```python
from build123d import *

# Parameters (mm, degrees)
SKETCH1_W                 = 25.4
SKETCH1_H                 = 15.24
BOSS_EXTRUDE1_DEPTH       = 0.79375
EDGE_FLANGE1_DEPTH        = 25.4
F_6_START                 = -0.79375
F_6_CLEARANCE_SLOT1_DEPTH = 1.5875
M18_CLEARANCE_HOLE1_D     = 20
M18_CLEARANCE_HOLE1_DEPTH = 9.652
M18_CLEARANCE_HOLE1_TIP   = 6.00860619


# Read off the part's stored shape, not the designer's step: #6 Clearance Slot1
# Sheet-metal steps are written as plain solids
with BuildPart() as part:
    # Sketch1 → Boss-Extrude1 (new, symmetric)
    with BuildSketch(Plane.XY):
        Rectangle(SKETCH1_W, SKETCH1_H)
    extrude(amount=BOSS_EXTRUDE1_DEPTH, both=True)

    # Edge-Flange1 section (across the edge) → Edge-Flange1 (add)
    with BuildSketch(Plane(origin=(-12.7, 7.988235857, -0.79375), x_dir=(0, -0.7071067811865438, -0.7071067811865512), z_dir=(1, 0, 0))):
        with BuildLine():
            Line((-1.5875, 0.368235857), (-1.5875, 30.48))
            Line((-1.5875, 30.48), (0, 30.48))
            Line((0, 30.48), (0, 0.368235857))
            ThreePointArc((0, 0.368235857), (0.067671096, 0.028030286), (0.260382072, -0.260382072))
            Line((0.260382072, -0.260382072), (-0.862149944, -1.382914087))
            ThreePointArc((-0.862149944, -1.382914087), (-1.398987662, -0.579479663), (-1.5875, 0.368235857))
        make_face()
    extrude(amount=EDGE_FLANGE1_DEPTH)

    # #6 Clearance Slot1 outline → #6 Clearance Slot1 (cut)
    with BuildSketch(Plane.XY.offset(F_6_START)):
        with BuildLine():
            ThreePointArc((-3.24485, 3.4925), (-5.3975, 5.64515), (-7.55015, 3.4925))
            Line((-7.55015, 3.4925), (-7.55015, -3.4925))
            ThreePointArc((-7.55015, -3.4925), (-5.3975, -5.64515), (-3.24485, -3.4925))
            Line((-3.24485, -3.4925), (-3.24485, 3.4925))
        make_face()
        with BuildLine():
            ThreePointArc((3.24485, -3.4925), (5.3975, -5.64515), (7.55015, -3.4925))
            Line((7.55015, -3.4925), (7.55015, 3.4925))
            ThreePointArc((7.55015, 3.4925), (5.3975, 5.64515), (3.24485, 3.4925))
            Line((3.24485, 3.4925), (3.24485, -3.4925))
        make_face()
    extrude(amount=F_6_CLEARANCE_SLOT1_DEPTH, mode=Mode.SUBTRACT)

    # M18 Clearance Hole1
    with Locations(Plane(origin=(0, 3.597242928, 3.597242928), x_dir=(-1, 0, 0), z_dir=(0, -0.7071067811865438, -0.7071067811865512))):
        with Locations((0, 21.818037609)):
            Hole(M18_CLEARANCE_HOLE1_D / 2, depth=M18_CLEARANCE_HOLE1_DEPTH)
            with Locations((0, 0, -(M18_CLEARANCE_HOLE1_DEPTH + M18_CLEARANCE_HOLE1_TIP / 2))):  # 118° drill point
                Cone(0, M18_CLEARANCE_HOLE1_D / 2, M18_CLEARANCE_HOLE1_TIP, mode=Mode.SUBTRACT)


solid = part.part
```
Geometry: final body of the model. Coordinates: model frame, mm. A direction names the side the tool comes from. Coordinates: 2 decimals unless noted, no trailing zeros. Write each loop counter-clockwise with the first axis right and the second up, starting at its lowest first coordinate (ties: lowest second). Pieces come first, ordered by that corner, then holes. Notation, with made-up numbers: M 52,-38 L 79,-38 A21 ccw 79,1 Z; hole C -2.5,39 d6. An arc over 180 degrees is marked long. Answer as CSV lines item,"result". Start each with the question number.
Q1. Pin query (flat end, axial travel): P1, Ø4, axis at x = 1, y = 14, coming from the -Z side; P2, Ø12, axis at y = 4.5, z = -1.5, coming from the -X side; P3, Ø6, axis at x = 8.5, y = 17.5, coming from the -Z side; P4, Ø4, axis at x = 6.5, y = -2, coming from the -Z side. Return the tip coordinate at first contact, or that it passes through.
Q2. Cut plane A-A on y = 3. Return the cut outline in (x, z).
Q3. Mould query, pull axis X, two halves, no side actions, for faces 1 (the flat face through (-3, 26.141, -18.947)), 2 (the flat face through (3.245, 0, 0)), 3 (the flat face through (-12.7, 14, -6)). Classes: released by +X, released by -X, zero draft, split by the parting line, or undercut.
Q4. Cut plane C-C on x = -9. Return the cut outline in (y, z), then the cut area to 3 significant figures.
Q5. Line query: line 1 (Z direction, x = -8.5, y = 0); line 2 (Z direction, x = 4.75, y = 9.5); line 3 (Y direction, x = 4.5, z = -18.75). Output: solid intervals per line, ascending. Write a range as from..to.
Q6. Reachability of faces 4 (the flat face through (0, 0, 0.794)), 5 (the flat face through (-3.245, 0, 0)), 6 (the flat face through (0, 0, -0.794)) from +Z, -Z, +X, -X, +Y, -Y: full face, straight path, thin tool, end or side. Return the list, or none.
Q7. Cut plane B-B on x = 11.25. Return the cut outline in (y, z), then the cut area to 3 significant figures.
Q8. Cut plane D-D on x = -5.25. Return the cut outline in (y, z), then the cut area to 3 significant figures.
Findings below:
1,P1,"stops at z = -4.81"
1,P2,"stops at x = -12.7"
1,P3,"stops at z = -12.98"
1,P4,"stops at z = -0.79"
2,outline,"M -12.7,-0.79 L -7.55,-0.79 L -7.55,0.79 L -12.7,0.79 Z; M -3.24,-0.79 L 3.24,-0.79 L 3.24,0.79 L -3.24,0.79 Z; M 7.55,-0.79 L 12.7,-0.79 L 12.7,0.79 L 7.55,0.79 Z"
3,face 1,"zero draft"
3,face 2,"undercut"
3,face 3,"released by -X"
4,outline,"M -7.62,-0.79 L 7.62,-0.79 A0.89 cw 8.25,-1.05 L 15.94,-8.75 L 17.07,-7.63 L 9.37,0.07 A2.48 ccw 7.62,0.79 L -7.62,0.79 Z; M 22.11,-14.91 L 29.54,-22.35 L 30.66,-21.22 L 23.23,-13.79 Z"
4,area,"60.3 mm2"
5,line 1,"z = -0.79..0.79"
5,line 2,"z = -2.31..-0.06"
5,line 3,"y = 25.94..28.19"
6,face 4,"+Z, +X, -X, +Y, -Y"
6,face 5,"+Z, -Z"
6,face 6,"-Z, +X, -X, -Y"
7,outline,"M -7.62,-0.79 L 7.62,-0.79 A0.89 cw 8.25,-1.05 L 29.54,-22.35 L 30.66,-21.22 L 9.37,0.07 A2.48 ccw 7.62,0.79 L -7.62,0.79 Z"
7,area,"74.1 mm2"
8,outline,"M -7.62,-0.79 L -5.64,-0.79 L -5.64,0.79 L -7.62,0.79 Z; M 5.64,-0.79 L 7.62,-0.79 A0.89 cw 8.25,-1.05 L 13.01,-5.81 L 14.13,-4.69 L 9.37,0.07 A2.48 ccw 7.62,0.79 L 5.64,0.79 Z; M 25.04,-17.85 L 29.54,-22.35 L 30.66,-21.22 L 26.17,-16.73 Z"
8,area,"29.2 mm2"
